Autodesk Inventor part; units mm, degrees
ref_plane "YZ Plane" through (0, 0, 0) normal (1, 0, 0) x (0, 1, 0)
ref_plane "XZ Plane" through (0, 0, 0) normal (0, 1, 0) x (-1, 0, 0)
ref_plane "XY Plane" through (0, 0, 0) normal (0, 0, 1) x (1, 0, 0)
sketch "Sketch1" plane through (0, 0, 0) normal (1, 0, 0) x (0, 1, 0)
  circle A0 centre (0, 0) radius 2.54
  circle A1 centre (0, 0) radius 6.35
  line L0 (0, 6.35) -> (40.2531, 6.35)
  line L1 (40.2531, 6.35) -> (40.2531, -6.35)
  line L2 (40.2531, -6.35) -> (0, -6.35)
  line L3 (40.2531, 6.35) -> (34.5987, -6.35)
  line L4 (35.1642, -5.08) -> (3.81, -5.08)
  line L5 (5.4993, 3.175) -> (10.2653, -5.08)
  line L6 (12.8053, -5.08) -> (12.8053, -6.35)
  dimension "d0" = 5.08
  dimension "d1" = 12.7
  dimension "d2" = 66
  dimension "d12" = 3.175
  dimension "d13" = 1.27
  dimension "d16" = 2.54
extrude "Extrusion1" add sketch "Sketch1" along normal mid plane 25.4 contours A1 | A1 L5 L4 | A1 L0 L3 L4 L5 | L4 L6 L2 A1 | L4 L3 L2 L6
chamfer "Chamfer1" distance 1.5875 distance2 3.175 1 edges at (0, 34.5987, -6.35) measured on face at (4.2333, 23.0658, -6.35)
chamfer "Chamfer2" distance 4.7625 distance2 1.5875 1 edges at (0, 40.2531, 6.35) measured on face at (4.2333, 38.7988, 3.0835)
fillet "Fillet1" radius 3.175 4 edges at (0, 38.6656, 6.35) (0, 38.316, 1.9992) (0, 35.8901, -3.4495) (0, 33.0112, -6.35)
extrude "Extrusion2" cut sketch "Sketch1" along normal mid plane 19.05 contours A1 L0 L3 L4 L5
extrude "Extrusion3" cut sketch "Sketch1" along normal mid plane 6.35 contours A1 | A1 L5 L4 | L4 L6 L2 A1
properties part number "LegV5"
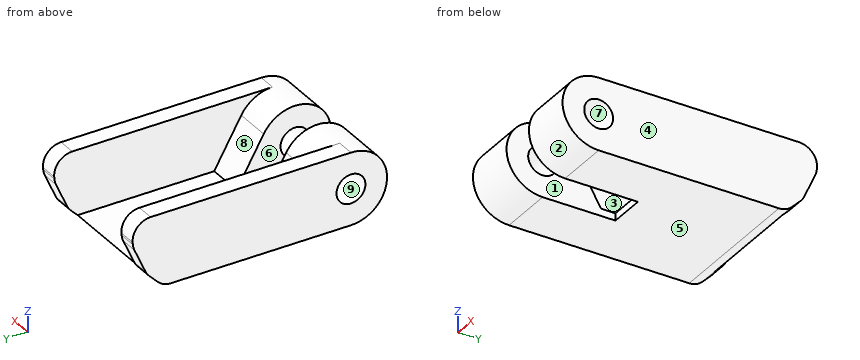
Here's how the part is built. I have some questions about the finished solid (model axes, mm). Face numbers are marked on the shaded views. A direction names the side the tool comes from. Round coordinates to 2 decimals unless told otherwise and drop trailing zeros. Loops run counter-clockwise (first coordinate to the right, second up) from the corner with the lowest first, then second, coordinate; pieces in that order, holes last.
1. If we section it at A-A on y = 23.5: Write out the boundary of the cut face in (x, z) (3 decimals).
Answer list:
outline: (-12.7, -6.35) - (12.7, -6.35) - (12.7, 6.35) - (9.525, 6.35) - (9.525, -5.08) - (-9.525, -5.08) - (-9.525, 6.35) - (-12.7, 6.35) - close
2. If I drill on line 1 along X through (y, z) = (34, 0.25) (3 decimals); line 2 along Z through (x, y) = (8.25, 0), over which ranges is the centre line in solid material (lowest first)?
Answer list:
line 1: x = -12.7 to -9.525, 9.525 to 12.7
line 2: z = -6.35 to -2.54, 2.54 to 6.35
3. We'd pull the mould along Z, two halves only. Please class the marked faces 6, 7, 8 and 9: +Z half, -Z half, draft (parallel to the pull), parting line (faces both ways), or undercut.
Answer list:
face 6: draft
face 7: undercut
face 8: +Z half
face 9: undercut
4. If we section it at D-D on z = -1: Write out the boundary of the cut face in (x, y) (3 decimals).
Answer list:
outline: (-12.7, -6.271) - (-3.175, -6.271) - (-3.175, -2.335) - (-12.7, -2.335) - close; (-12.7, 2.335) - (-3.175, 2.335) - (-3.175, 7.91) - (-9.525, 7.91) - (-9.525, 36.981) - (-12.7, 36.981) - close; (3.175, -6.271) - (12.7, -6.271) - (12.7, -2.335) - (3.175, -2.335) - close; (3.175, 2.335) - (12.7, 2.335) - (12.7, 36.981) - (9.525, 36.981) - (9.525, 7.91) - (3.175, 7.91) - close
5. For P1, Ø2, axis at x = 5.5, z = 1.5, coming from the +Y side; P2, Ø8, axis at x = -3, y = 14, coming from the +Z side; P3, Ø2, axis at x = -7, z = 0.5, coming from the -Y side; P4, Ø1.4, axis at x = 1.5, z = -5.5, coming from the -Y side, each with a flat end and sliding along its axis, tell me the tip position at first contact or that it passes through.
Answer list:
P1: stops at y = 7.04
P2: stops at z = -4.63
P3: stops at y = -6.35
P4: stops at y = 12.81
6. If we section it at C-C on x = 8.25: Write out the boundary of the cut face in (y, z) (3 decimals).
Answer list:
outline: (0, -6.35) - (31.689, -6.35) arc R3.175 ccw to (33.943, -5.412) - (34.272, -5.08) - (10.265, -5.08) - (5.499, 3.175) arc R6.35 ccw (long way) to start; hole circle Ø5.08 at (0, 0)
7. If we section it at B-B on y = 1.5: Write out the boundary of the cut face in (x, z) (3 decimals), plus the area to 3 significant figures.
Answer list:
outline: (-12.7, -6.35) - (-3.175, -6.35) - (-3.175, -2.05) - (-12.7, -2.05) - close; (-12.7, 2.05) - (-3.175, 2.05) - (-3.175, 6.17) - (-9.525, 6.17) - (-9.525, 6.35) - (-12.7, 6.35) - close; (3.175, -6.35) - (12.7, -6.35) - (12.7, -2.05) - (3.175, -2.05) - close; (3.175, 2.05) - (12.7, 2.05) - (12.7, 6.35) - (9.525, 6.35) - (9.525, 6.17) - (3.175, 6.17) - close
area: 162 mm2
8. Which directions (+Z, -Z, +X, -X, +Y, -Y) give clear straight access to the entire face, cutting with the end or side of a thin tool? Please do the marked faces 1, 2, 3, 4 and 5.
Answer list:
face 1: +Z, -Z, -Y
face 2: none
face 3: +Z, +Y
face 4: +Z, -Z, +X, +Y, -Y
face 5: -Z, +X, -X, +Y, -Y
